The listing builds one solid part. Answer for the finished solid, in the listing's coordinates (mm). A direction names the side the tool comes from. Give positions to 0.01 mm unless a question says otherwise; leave off trailing zeros. Loops run counter-clockwise (first coordinate to the right, second up) from the corner with the lowest first, then second, coordinate; pieces in that order, holes last.
Item 1: Each of these flat-tipped pins is pushed along its axis until it touches: pin 1 Ø3.5 at (x, z) = (-47, 1.75) entering from +Y (3 decimals); pin 2 Ø6.5 at (x, y) = (4, 1.5) entering from +Z; pin 3 Ø2.5 at (y, z) = (1, 8.5) entering from +X; pin 4 Ø1.8 at (x, z) = (-47, 8.25) entering from +Y (3 decimals). Where does it stop, or does it pass through?
Item 2: A tool of negligible diameter and unlimited length cuts with its end or side. For faces 4 (the face through (44, -2.925, 5)), 5 (the face through (42.25, 4.28, 4.93)), 6 (the face through (-48.5, 0, 7)), 7 (the face through (38, 0, 3)), from which of +Z, -Z, +X, -X, +Y, -Y can it reach the whole face along a straight path? Write none if from no direction.
Item 3: Section C-C, the plane x = 43.75 is taken. Give the vertices of the cut face in (y, z) (3 decimals), and give its area (3 significant figures).
Item 4: The mould has two halves that part along Z. Classify faces 1 (the face through (45.5, 4.3, 1.7)), 2 (the face through (44, 0, 1)), 3 (the face through (50, -1, 2)): pulls with the +Z half, pulls with the -Z half, needs draft (parallel to the pull), parting line crosses it, or undercut.
Item 5: Consider line 1 along Z through (x, y) = (-47, 4.5); line 2 along X through (y, z) = (-3.8, 1.75); line 3 along Y through (x, z) = (-14, 8.5) (3 decimals). Determine where each line is inside the solid, lowest interval first.
Item 6: Section B-B, the plane y = 1.5 is taken. Give the vertices of the cut face in (x, z).
Item 7: Section A-A, the plane x = -43.75 is taken. Give the vertices of the cut face in (y, z) (3 decimals), and give its area (3 significant figures).
from build123d import *

# Parameters (mm, degrees)
ESBO_O1_W                = 5
ESBO_O1_H                = 5.35
RESSALTO_EXTRUS_O1_DEPTH = 50
CORTE_EXTRUS_O5_START    = -2.675
CORTE_EXTRUS_O5_DEPTH    = 5.35
FILETE2_R                = 2
SKETCH1_W                = 100
SKETCH1_H                = 10
BOSS_EXTRUDE1_DEPTH      = 3
SKETCH2_W                = 100
SKETCH2_H                = 20
BOSS_EXTRUDE2_DEPTH      = 3
FILLET1_R                = 2
FILLET2_R                = 2
CUT_EXTRUDE1_START       = 2.925
CUT_EXTRUDE1_OUTLINE_R   = 1.5
CUT_EXTRUDE1_DEPTH       = 2.75
SKETCH6_W                = 5
SKETCH6_H                = 5.35
BOSS_EXTRUDE4_DEPTH      = 1.5
SKETCH8_R                = 1.5
CUT_EXTRUDE2_DEPTH       = 2.75
CHAMFER2_SIZE            = 1.25
CUT_EXTRUDE3_DEPTH       = 10
FILLET3_R                = 10
FILLET4_R                = 5


# Read off the part's stored shape, not the designer's step: Corte-extrusão5, Cut-Extrude1
with BuildPart() as part:
    # Esboço1 → Ressalto-extrusão1 (new, symmetric)
    with BuildSketch(Plane(origin=(0, 0, 0), x_dir=(0, 0, -1), z_dir=(1, 0, 0))):
        with Locations((-2.5, 0)):
            Rectangle(ESBO_O1_W, ESBO_O1_H)
    extrude(amount=RESSALTO_EXTRUS_O1_DEPTH, both=True)

    # Corte-extrusão5 outline → Corte-extrusão5 (cut)
    with BuildSketch(Plane(origin=(0, 0, 0), x_dir=(1, 0, 0), z_dir=(0, 1, 0)).offset(CORTE_EXTRUS_O5_START)):
        Polygon((46, -5), (45, -0.2), (33, -5), align=None)
    extrude(amount=CORTE_EXTRUS_O5_DEPTH, mode=Mode.SUBTRACT)

    # Filete2
    filete2_edges = [part.edges().sort_by_distance(p)[0] for p in [
        (46, 0, 5),
    ]]
    fillet(filete2_edges, radius=FILETE2_R)

    # Sketch1 → Boss-Extrude1 (add)
    with BuildSketch(Plane(origin=(0, 2.675, 0), x_dir=(1, 0, 0), z_dir=(0, 1, 0))):
        with Locations((0, -5)):
            Rectangle(SKETCH1_W, SKETCH1_H)
    extrude(amount=BOSS_EXTRUDE1_DEPTH)

    # Sketch2 → Boss-Extrude2 (add)
    with BuildSketch(Plane.XZ.offset(2.675)):
        with Locations((0, 10)):
            Rectangle(SKETCH2_W, SKETCH2_H)
    extrude(amount=BOSS_EXTRUDE2_DEPTH)

    # Fillet1
    fillet1_edges = [part.edges().sort_by_distance(p)[0] for p in [
        (45, 0, 0.2),
    ]]
    fillet(fillet1_edges, radius=FILLET1_R)

    # Fillet2
    fillet2_edges = [part.edges().sort_by_distance(p)[0] for p in [
        (33, 0, 5),
    ]]
    fillet(fillet2_edges, radius=FILLET2_R)

    # Cut-Extrude1 outline → Cut-Extrude1 (cut)
    with BuildSketch(Plane(origin=(0, 0, 0), x_dir=(1, 0, 0), z_dir=(0, 1, 0)).offset(CUT_EXTRUDE1_START)):
        with Locations((-43.75, -5)):
            Circle(CUT_EXTRUDE1_OUTLINE_R)
        with Locations((43.75, -5)):
            Circle(CUT_EXTRUDE1_OUTLINE_R)
        with Locations((47, -1.75)):
            Circle(CUT_EXTRUDE1_OUTLINE_R)
        with Locations((47, -8.25)):
            Circle(CUT_EXTRUDE1_OUTLINE_R)
        with Locations((-47, -8.25)):
            Circle(CUT_EXTRUDE1_OUTLINE_R)
        with Locations((-47, -1.75)):
            Circle(CUT_EXTRUDE1_OUTLINE_R)
    extrude(amount=CUT_EXTRUDE1_DEPTH, mode=Mode.SUBTRACT)

    # Sketch6 → Boss-Extrude4 (add)
    with BuildSketch(Plane.ZY.offset(50)):
        with Locations((7.5, 0)):
            Rectangle(SKETCH6_W, SKETCH6_H)
    extrude(amount=-BOSS_EXTRUDE4_DEPTH)

    # Sketch8 → Cut-Extrude2 (cut)
    with BuildSketch(Plane.XZ.offset(5.675)):
        with Locations(Location((47, 8.25, 0), (0, 0, 90))):
            Circle(SKETCH8_R)
        with Locations(Location((43.75, 5, 0), (0, 0, 270))):
            Circle(SKETCH8_R)
        with Locations(Location((47, 1.75, 0), (0, 0, 270))):
            Circle(SKETCH8_R)
        with Locations(Location((-47, 8.25, 0), (0, 0, 270))):
            Circle(SKETCH8_R)
        with Locations(Location((-43.75, 5, 0), (0, 0, 90))):
            Circle(SKETCH8_R)
        with Locations(Location((-47, 1.75, 0), (0, 0, 90))):
            Circle(SKETCH8_R)
    extrude(amount=-CUT_EXTRUDE2_DEPTH, mode=Mode.SUBTRACT)

    # Chamfer2
    chamfer2_edges = [part.edges().sort_by_distance(p)[0] for p in [
        (50, 2.675, 7.5),
        (50, 0, 5),
    ]]
    chamfer(chamfer2_edges, length=CHAMFER2_SIZE)

    # Sketch10 → Cut-Extrude3 (cut)
    with BuildSketch(Plane(origin=(0, -2.675, 0), x_dir=(1, 0, 0), z_dir=(0, 1, 0))):
        with BuildLine():
            Line((-37.586485056, -20), (37.586485056, -20))
            add(Edge.make_bspline(
                [(37.586485056, -20), (27.768328162, -9.955951582), (0, -9.955951582)],
                knots=[0, 0, 0, 1, 1, 1], degree=2))
            add(Edge.make_bspline(
                [(-37.586485056, -20), (-27.768328162, -9.955951582), (0, -9.955951582)],
                knots=[0, 0, 0, 1, 1, 1], degree=2))
        make_face()
    extrude(amount=-CUT_EXTRUDE3_DEPTH, mode=Mode.SUBTRACT)

    # Fillet3
    fillet3_edges = [part.edges().sort_by_distance(p)[0] for p in [
        (37.586485056, -4.175, 20),
        (-37.586485056, -4.175, 20),
    ]]
    fillet(fillet3_edges, radius=FILLET3_R)

    # Fillet4
    fillet4_edges = [part.edges().sort_by_distance(p)[0] for p in [
        (-50, -4.175, 20),
        (50, -4.175, 20),
    ]]
    fillet(fillet4_edges, radius=FILLET4_R)


solid = part.part
Worked answers:
1. pin 1: stops at y = 5.675
1. pin 2: stops at z = 10
1. pin 3: stops at x = -48.5
1. pin 4: stops at y = 2.925
2. face 4: -Y
2. face 5: +Y
2. face 6: +Z, +X
2. face 7: +Z
3. outline: (-5.675, 0) - (5.675, 0) - (5.675, 3.5) - (2.925, 3.5) - (2.925, 6.5) - (5.675, 6.5) - (5.675, 10) - (2.675, 10) - (2.675, 0.955) - (-2.675, 0.955) - (-2.675, 20) - (-5.675, 20) - (-5.675, 6.5) - (-2.925, 6.5) - (-2.925, 3.5) - (-5.675, 3.5) - close
3. area: 78.6 mm2
4. face 1: undercut
4. face 2: pulls with the +Z half
4. face 3: needs draft
5. line 1: z = 0 to 0.25, 3.25 to 6.75, 9.75 to 10
5. line 2: x = -50 to -48.5, -45.5 to 45.5, 48.5 to 50
5. line 3: y = -5.675 to -2.675, 2.675 to 5.675
6. outline: (-50, 0) - (50, 0) - (50, 3.75) - (48.75, 5) - (47.63, 5) arc R2 ccw to (45.67, 3.41) - (45.49, 2.53) arc R2 cw to (42.79, 1.09) - (33.36, 4.86) arc R2 ccw to (32.61, 5) - (-48.5, 5) - (-48.5, 10) - (-50, 10) - close
7. outline: (-5.675, 0) - (5.675, 0) - (5.675, 3.5) - (2.925, 3.5) - (2.925, 6.5) - (5.675, 6.5) - (5.675, 10) - (2.675, 10) - (2.675, 5) - (-2.675, 5) - (-2.675, 20) - (-5.675, 20) - (-5.675, 6.5) - (-2.925, 6.5) - (-2.925, 3.5) - (-5.675, 3.5) - close
7. area: 100 mm2
